Could you check a few things on this model? Use its own coordinates, in mm. Round coordinates to 2 decimals unless told otherwise and drop trailing zeros. Order: outer loops, then holes, each group sorted by start corner. A loop starts at its lowest first (then second) coordinate and runs counter-clockwise, first axis right, second up. Notation, with made-up numbers: M 54,-26.5 L 66,-26.5 A23 ccw 66,-17.5 Z; hole C -3,88.25 d9. An arc over 180 degrees is marked long. Write each question's results on one line, items separated by ' | '. Start each with the question number.
1. We'd pull the mould along X, two halves only. Please class faces 1 (the cylindrical face through (12.344, 0.173, 0.145)), 2 (the cylindrical face through (8.001, 0.173, -6.316)), 3 (the cylindrical face through (-8.417, 0.173, -6.664)), 4 (the flat face through (5.3, 0, 5.3)): released by +X, released by -X, zero draft, split by the parting line, or undercut.
2. Suppose I cut it at D-D on y = 0.2. Write out the boundary of the cut face in (x, z), and give its area (3 significant figures).
3. Suppose I cut it at B-B on z = 0. Write out the boundary of the cut face in (x, y).
4. Suppose I cut it at C-C on x = -6.5. Write out the boundary of the cut face in (y, z).
5. I'm going to push a flat-ended pin straight in: pin 1 (1.5 mm diameter, centred on x = -7.42, z = 7.42, fed in from -Y). Where does the tip first touch, or does it pass through?
6. Please list where these lines run through material, in increasing order: L1, parallel to X at y = 0.1, z = 0; L2, parallel to X at y = 0.1, z = 2.25.
7. Suppose I cut it at A-A on x = 0. Write out the boundary of the cut face in (y, z), and give its area (3 significant figures).
from build123d import *

# Parameters (mm, degrees)
SKETCH1_R           = 7.25
SKETCH1_R_2         = 1.25
BOSS_EXTRUDE1_DEPTH = 0.35


with BuildPart() as part:
    # Sketch1 → Boss-Extrude1 (new body)
    with BuildSketch(Plane(origin=(0, 0, 0), x_dir=(1, 0, 0), z_dir=(0, 1, 0))):
        with BuildLine():
            ThreePointArc((10, -10), (12.344355629, 0), (10, 10))
            ThreePointArc((10, 10), (0, 12.344355629), (-10, 10))
            ThreePointArc((-10, 10), (-12.344355629, 0), (-10, -10))
            ThreePointArc((-10, -10), (0, -12.344355629), (10, -10))
        make_face()
        Circle(SKETCH1_R, mode=Mode.SUBTRACT)
        with Locations((7.424621202, 7.424621202)):
            Circle(SKETCH1_R_2, mode=Mode.SUBTRACT)
        with Locations((7.424621202, -7.424621202)):
            Circle(SKETCH1_R_2, mode=Mode.SUBTRACT)
        with Locations((-7.424621202, -7.424621202)):
            Circle(SKETCH1_R_2, mode=Mode.SUBTRACT)
        with Locations((-7.424621202, 7.424621202)):
            Circle(SKETCH1_R_2, mode=Mode.SUBTRACT)
    extrude(amount=BOSS_EXTRUDE1_DEPTH)


solid = part.part
Filled sheet:
1) face 1: released by +X | face 2: undercut | face 3: undercut | face 4: zero draft
2) outline: M -10,-10 A22.5 ccw 10,-10 A22.5 ccw 10,10 A22.5 ccw -10,10 A22.5 ccw Z; hole C -7.42,-7.42 d2.5; hole C -7.42,7.42 d2.5; hole C 0,0 d14.5; hole C 7.42,-7.42 d2.5; hole C 7.42,7.42 d2.5 | area: 342 mm^2
3) outline: M -12.34,0 L -7.25,0 L -7.25,0.35 L -12.34,0.35 Z; M 7.25,0 L 12.34,0 L 12.34,0.35 L 7.25,0.35 Z
4) outline: M 0,-11.39 L 0.35,-11.39 L 0.35,-8.27 L 0,-8.27 Z; M 0,-6.58 L 0.35,-6.58 L 0.35,-3.21 L 0,-3.21 Z; M 0,3.21 L 0.35,3.21 L 0.35,6.58 L 0,6.58 Z; M 0,8.27 L 0.35,8.27 L 0.35,11.39 L 0,11.39 Z
5) pin 1: passes through
6) L1: x = -12.34 to -7.25, 7.25 to 12.34 | L2: x = -12.23 to -6.89, 6.89 to 12.23
7) outline: M 0,-12.34 L 0.35,-12.34 L 0.35,-7.25 L 0,-7.25 Z; M 0,7.25 L 0.35,7.25 L 0.35,12.34 L 0,12.34 Z | area: 3.57 mm^2
